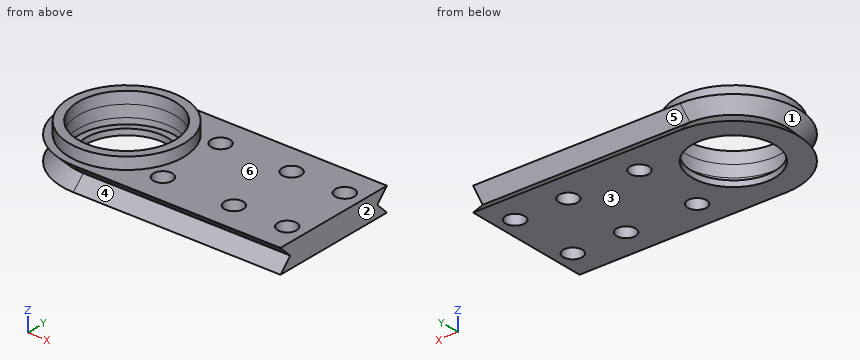
from build123d import *

# Parameters (mm, degrees)
PAD_DEPTH            = 35
SKETCH004_R          = 1.6
POCKET_DEPTH         = 2.001
POCKET_DEPTH_BACK    = 2.001
SKETCH006_R          = 7
POCKET001_DEPTH      = 2.001
POCKET001_DEPTH_BACK = 2.001
SKETCH005_R          = 8.15
POCKET002_DEPTH      = 1
POCKET002_DEPTH_BACK = 100
SKETCH007_R          = 9.65
SKETCH007_R_2        = 8.15
PAD001_DEPTH         = 2


with BuildPart() as part:
    # Sketch → Pad (new body)
    with BuildSketch(Plane.YZ):
        Polygon((0, 2), (-10.9, 2), (-8.9, 0), (-10.9, -2), (0, -2), (10.9, -2), (8.9, 0), (10.9, 2), align=None)
    extrude(amount=PAD_DEPTH)

    # Sketch002 (on DatumPlane) → AdditiveLoft section 0
    with BuildSketch(Plane.XY.offset(2)):
        with BuildLine():
            ThreePointArc((0, 10.9), (-10.9, 0), (0, -10.9))
            Line((0, 10.9), (0, -10.9))
        make_face()
    # Sketch001 → AdditiveLoft section 1
    with BuildSketch(Plane.XY):
        with BuildLine():
            ThreePointArc((0, 8.9), (-8.9, 0), (0, -8.9))
            Line((0, 8.9), (0, -8.9))
        make_face()
    # Sketch003 (on DatumPlane) → AdditiveLoft section 2
    with BuildSketch(Plane.XY.offset(-2)):
        with BuildLine():
            ThreePointArc((0, 10.9), (-10.9, 0), (0, -10.9))
            Line((0, 10.9), (0, -10.9))
        make_face()
    loft(ruled=True)

    # Sketch004 → Pocket (cut, two sides)
    with BuildSketch(Plane.XY) as pocket_sk:
        with Locations((32, 5.9)):
            Circle(SKETCH004_R)
        with Locations((32, -5.9)):
            Circle(SKETCH004_R)
        with Locations((23, 5.9)):
            Circle(SKETCH004_R)
        with Locations((11, 5.9)):
            Circle(SKETCH004_R)
        with Locations((23, -5.9)):
            Circle(SKETCH004_R)
        with Locations((11, -5.9)):
            Circle(SKETCH004_R)
    extrude(amount=-POCKET_DEPTH, mode=Mode.SUBTRACT)
    extrude(pocket_sk.sketch, amount=POCKET_DEPTH_BACK, mode=Mode.SUBTRACT)

    # Sketch006 → Pocket001 (cut, two sides)
    with BuildSketch(Plane.XY) as pocket001_sk:
        Circle(SKETCH006_R)
    extrude(amount=-POCKET001_DEPTH, mode=Mode.SUBTRACT)
    extrude(pocket001_sk.sketch, amount=POCKET001_DEPTH_BACK, mode=Mode.SUBTRACT)

    # Sketch005 → Pocket002 (cut, two sides)
    with BuildSketch(Plane.XY) as pocket002_sk:
        Circle(SKETCH005_R)
    extrude(amount=-POCKET002_DEPTH, mode=Mode.SUBTRACT)
    extrude(pocket002_sk.sketch, amount=POCKET002_DEPTH_BACK, mode=Mode.SUBTRACT)

    # Sketch007 (on DatumPlane) → Pad001 (join)
    with BuildSketch(Plane.XY.offset(2)):
        Circle(SKETCH007_R)
        Circle(SKETCH007_R_2, mode=Mode.SUBTRACT)
    extrude(amount=PAD001_DEPTH)


solid = part.part
Build history of the part. All positions in model axes, mm. Face numbers are marked on the shaded views. A direction names the side the tool comes from. Give positions to 0.01 mm unless a question says otherwise; leave off trailing zeros. Order: outer loops, then holes, each group sorted by start corner. A loop starts at its lowest first (then second) coordinate and runs counter-clockwise, first axis right, second up. Notation, with made-up numbers: M 56.5,48 L 70.5,48 A22 cw 70.5,77 Z; hole C 63,46 d6. An arc over 180 degrees is marked long. Put each result on its own line as item: value.
Item 1: Cut at A-A on y = 0. Write the cut outline in (x, z).
Results are:
outline: M -10.9,-2 L -7,-2 L -7,-1 L -8.15,-1 L -8.15,4 L -9.65,4 L -9.65,2 L -10.9,2 L -8.9,0 Z; M 7,-2 L 35,-2 L 35,2 L 9.65,2 L 9.65,4 L 8.15,4 L 8.15,-1 L 7,-1 Z
Item 2: Cut at C-C on x = 19.5. Write the cut outline in (y, z).
Results are:
outline: M -10.9,-2 L 10.9,-2 L 8.9,0 L 10.9,2 L -10.9,2 L -8.9,0 Z
Item 3: Cut at B-B on x = 11. Write the cut outline in (y, z).
Results are:
outline: M -10.9,-2 L -7.5,-2 L -7.5,2 L -10.9,2 L -8.9,0 Z; M -4.3,-2 L 4.3,-2 L 4.3,2 L -4.3,2 Z; M 7.5,-2 L 10.9,-2 L 8.9,0 L 10.9,2 L 7.5,2 Z
Item 4: Which spindle directions (+Z, -Z, +X, -X, +Y, -Y) get a long thin tool onto all of the face, cutting with end or side? Do the marked faces 1 and 2. Say none if no direction does.
Results are:
face 1: -X
face 2: +Z, -Z, +X, +Y, -Y
Item 5: Cut at D-D on z = 3.45. Write the cut outline in (x, y), then the cut area to 3 significant figures.
Results are:
outline: C 0,0 d19.3; hole C 0,0 d16.3
area: 83.9 mm2
Item 6: Drop flat-ended pins along their axis: pin 1 Ø3 at (x, z) = (-4, -0.5) entering from +Y; pin 2 Ø1.5 at (y, z) = (-7, -1) entering from -X; pin 3 Ø4 at (x, y) = (11, -5.9) entering from +Z. Give the stop position or say it passes through.
Results are:
pin 1: y = 10.23
pin 2: x = -8.21
pin 3: z = 2
Item 7: Wall check: probe 1 along X at (y, z) = (-5.9, 1.25); probe 2 along Y at (x, z) = (32, -0.75); probe 3 along Y at (x, z) = (32, 1.55). Give the ranges that are in metal, low to high.
Results are:
probe 1: -8.26 to -5.62, 5.62 to 9.4, 12.6 to 21.4, 24.6 to 30.4, 33.6 to 35
probe 2: -9.65 to -7.5, -4.3 to 4.3, 7.5 to 9.65
probe 3: -10.45 to -7.5, -4.3 to 4.3, 7.5 to 10.45
Item 8: Pull direction Z, two halves, no side cores. Call the marked faces 3, 4, 5 and 6: +Z half, -Z half, draft (parallel to the pull), parting line (faces both ways), or undercut.
Results are:
face 3: -Z half
face 4: undercut
face 5: undercut
face 6: +Z half
